Could you check a few things on this model? Use its own coordinates, in mm. Give positions to 0.01 mm unless a question says otherwise; leave off trailing zeros. Order: outer loops, then holes, each group sorted by start corner. A loop starts at its lowest first (then second) coordinate and runs counter-clockwise, first axis right, second up.
(1) If we mould it in two halves opening along X, with no side actions, what happens to faces 1 (the cylindrical face through (35.09, 1.61, -35.25)), 2 (the cylindrical face through (-4.879, 1.61, 1.952)), 3 (the cylindrical face through (2.86, 1.61, 1.22)), 4 (the cylindrical face through (-35.25, 1.61, -35.09))? For each: released by +X, released by -X, zero draft, split by the parting line, or undercut.
(2) Imagine slicing it at C-C, the plane x = 3.5. Write out the boundary of the cut face in (y, z) (3 decimals).
(3) Imagine slicing it at A-A, the plane y = 1.5. Write out the boundary of the cut face in (x, z) (3 decimals), then the cut area to 3 significant figures.
(4) Will this pin go through, and if not, where does the flat tip stop? pin 1 (3 mm diameter, centred on x = -4.445, z = 0, fed in from +Y) (3 decimals).
(5) If I drill on probe 1 along X at (y, z) = (2.05, 0) (3 decimals); probe 2 along Z at (x, y) = (28.5, 2.3); probe 3 along Z at (x, y) = (-4, 0.65), over which ranges is the centre line in solid material (lowest first)?
(6) Imagine slicing it at B-B, the plane z = 0. Write out the boundary of the cut face in (x, y) (3 decimals), then the cut area to 3 significant figures.
from build123d import *

# Parameters (mm, degrees)
SKETCH1_W           = 76.2
SKETCH1_H           = 76.2
BOSS_EXTRUDE1_DEPTH = 3.175
FILLET1_R           = 10
FILLET2_R           = 10
FILLET3_R           = 10
FILLET4_R           = 10
SKETCH2_R           = 2
CUT_EXTRUDE1_DEPTH  = 4.175


with BuildPart() as part:
    # Sketch1 → Boss-Extrude1 (new body)
    with BuildSketch(Plane(origin=(0, 0, 0), x_dir=(1, 0, 0), z_dir=(0, 1, 0))):
        Rectangle(SKETCH1_W, SKETCH1_H)
    extrude(amount=BOSS_EXTRUDE1_DEPTH)

    # Fillet1
    fillet1_edges = [part.edges().sort_by_distance(p)[0] for p in [
        (-38.1, 1.5875, 38.1),
    ]]
    fillet(fillet1_edges, radius=FILLET1_R)

    # Fillet2
    fillet2_edges = [part.edges().sort_by_distance(p)[0] for p in [
        (-38.1, 1.5875, -38.1),
    ]]
    fillet(fillet2_edges, radius=FILLET2_R)

    # Fillet3
    fillet3_edges = [part.edges().sort_by_distance(p)[0] for p in [
        (38.1, 1.5875, -38.1),
    ]]
    fillet(fillet3_edges, radius=FILLET3_R)

    # Fillet4
    fillet4_edges = [part.edges().sort_by_distance(p)[0] for p in [
        (38.1, 1.5875, 38.1),
    ]]
    fillet(fillet4_edges, radius=FILLET4_R)

    # Sketch2 → Cut-Extrude1 (cut, through all)
    with BuildSketch(Plane(origin=(0, 3.175, 0), x_dir=(1, 0, 0), z_dir=(0, 1, 0))):
        with Locations((4.445, 0)):
            Circle(SKETCH2_R)
        with Locations((-4.445, 0)):
            Circle(SKETCH2_R)
    extrude(amount=-CUT_EXTRUDE1_DEPTH, mode=Mode.SUBTRACT)


solid = part.part
Answer block:
1. face 1: released by +X
1. face 2: undercut
1. face 3: undercut
1. face 4: released by -X
2. outline: (0, -38.1) - (3.175, -38.1) - (3.175, -1.763) - (0, -1.763) - close; (0, 1.763) - (3.175, 1.763) - (3.175, 38.1) - (0, 38.1) - close
3. outline: (-38.1, -28.1) arc R10 ccw to (-28.1, -38.1) - (28.1, -38.1) arc R10 ccw to (38.1, -28.1) - (38.1, 28.1) arc R10 ccw to (28.1, 38.1) - (-28.1, 38.1) arc R10 ccw to (-38.1, 28.1) - close; hole circle Ø4 at (-4.445, 0); hole circle Ø4 at (4.445, 0)
3. area: 5,700 mm2
4. pin 1: passes through
5. probe 1: x = -38.1 to -6.445, -2.445 to 2.445, 6.445 to 38.1
5. probe 2: z = -38.09 to 38.09
5. probe 3: z = -38.1 to -1.95, 1.95 to 38.1
6. outline: (-38.1, 0) - (-6.445, 0) - (-6.445, 3.175) - (-38.1, 3.175) - close; (-2.445, 0) - (2.445, 0) - (2.445, 3.175) - (-2.445, 3.175) - close; (6.445, 0) - (38.1, 0) - (38.1, 3.175) - (6.445, 3.175) - close
6. area: 217 mm2
